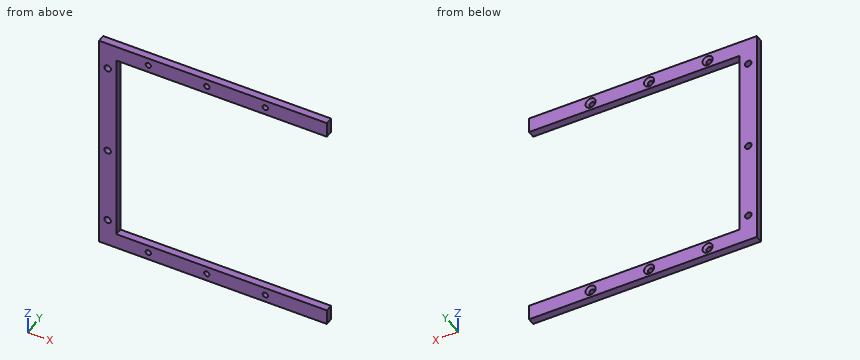
```python
from build123d import *

# Parameters (mm, degrees)
SKETCH2_W           = 7.119984
SKETCH2_H           = 81.28
SKETCH2_R           = 1.35
SKETCH2_W_2         = 93.98
SKETCH2_H_2         = 6.35
SKETCH2_R_2         = 1.1
BOSS_EXTRUDE1_DEPTH = 3
CHAMFER1_SIZE       = 1


with BuildPart() as part:
    # Sketch2 → Boss-Extrude1 (new body)
    # profile 1 of 3: a face of its own
    with BuildSketch(Plane(origin=(0, 0, 0), x_dir=(1, 0, 0), z_dir=(0, 1, 0))):
        with Locations((3.559992, -46.99)):
            Rectangle(SKETCH2_W, SKETCH2_H)
        with Locations(Location((3.559992, -82.490012, 0), (0, 0, 270))):
            Circle(SKETCH2_R, mode=Mode.SUBTRACT)
        with Locations(Location((3.559992, -43.990012, 0), (0, 0, 270))):
            Circle(SKETCH2_R, mode=Mode.SUBTRACT)
        with Locations(Location((3.559992, -11.490012, 0), (0, 0, 270))):
            Circle(SKETCH2_R, mode=Mode.SUBTRACT)
    # profile 2 of 3: a face of its own
    with BuildSketch(Plane(origin=(0, 0, 0), x_dir=(1, 0, 0), z_dir=(0, 1, 0))):
        with Locations((46.99, -3.175)):
            Rectangle(SKETCH2_W_2, SKETCH2_H_2)
        with Locations(Location((68.58, -3.155, 0), (0, 0, 270))):
            Circle(SKETCH2_R_2, mode=Mode.SUBTRACT)
        with Locations(Location((44.45, -3.155, 0), (0, 0, 270))):
            Circle(SKETCH2_R_2, mode=Mode.SUBTRACT)
        with Locations(Location((20.32, -3.155, 0), (0, 0, 270))):
            Circle(SKETCH2_R_2, mode=Mode.SUBTRACT)
    # profile 3 of 3: a face of its own
    with BuildSketch(Plane(origin=(0, 0, 0), x_dir=(1, 0, 0), z_dir=(0, 1, 0))):
        with Locations((46.99, -90.805)):
            Rectangle(SKETCH2_W_2, SKETCH2_H_2)
        with Locations(Location((68.58, -90.805, 0), (0, 0, 270))):
            Circle(SKETCH2_R_2, mode=Mode.SUBTRACT)
        with Locations(Location((44.45, -90.805, 0), (0, 0, 270))):
            Circle(SKETCH2_R_2, mode=Mode.SUBTRACT)
        with Locations(Location((20.32, -90.805, 0), (0, 0, 270))):
            Circle(SKETCH2_R_2, mode=Mode.SUBTRACT)
    extrude(amount=BOSS_EXTRUDE1_DEPTH)

    # Chamfer1
    chamfer1_edges = [part.edges().sort_by_distance(p)[0] for p in [
        (20.32, 3, 89.705),
        (68.58, 3, 2.055),
        (44.45, 3, 2.055),
        (20.32, 3, 2.055),
        (68.58, 3, 89.705),
        (44.45, 3, 89.705),
    ]]
    chamfer(chamfer1_edges, length=CHAMFER1_SIZE)


solid = part.part
```
Design review of the part built by this model. Coordinates are the model's own, in mm. Coordinates: 2 decimals unless noted, no trailing zeros. Order: outer loops, then holes, each group sorted by start corner. A loop starts at its lowest first (then second) coordinate and runs counter-clockwise, first axis right, second up.
1) Take a section at C-C, the plane x = 20.32. Give the boundary of the cut face in (y, z) (3 decimals), and give its area (3 significant figures).
2) Clearance check with flat-ended pins moving along their axes: pin 1 (1.3 mm diameter, centred on x = 44.45, z = 3.155, fed in from +Y); pin 2 (1 mm diameter, centred on y = 2, z = 36.5, fed in from +X). State where each tip first meets the part, or that it passes through.
3) Take a section at B-B, the plane y = 1.15. State how many separate pieces and enclosed holes the cut face has, and give its area (3 significant figures).
4) Wall thickness on line 1 along Z through (x, y) = (68.58, 0.7) (3 decimals); line 2 along Z through (x, y) = (64, 0.2); line 3 along X through (y, z) = (0.95, 50): over which ranges is each line inside the solid? List them lowest first.
5) Take a section at D-D, the plane z = 73. Give the boundary of the cut face in (x, y).
6) Take a section at A-A, the plane x = 52.5. Give the boundary of the cut face in (y, z), and give its area (3 significant figures).
Returned:
1. outline: (0, 0) - (3, 0) - (3, 1.055) - (2, 2.055) - (0, 2.055) - close; (0, 4.255) - (2, 4.255) - (3, 5.255) - (3, 6.35) - (0, 6.35) - close; (0, 87.63) - (3, 87.63) - (3, 88.705) - (2, 89.705) - (0, 89.705) - close; (0, 91.905) - (2, 91.905) - (3, 92.905) - (3, 93.98) - (0, 93.98) - close
1. area: 22.9 mm2
2. pin 1: passes through
2. pin 2: stops at x = 7.12
3. separate pieces: 1
3. enclosed holes: 9
3. area: 1,730 mm2
4. line 1: z = 0 to 2.055, 4.255 to 6.35, 87.63 to 89.705, 91.905 to 93.98
4. line 2: z = 0 to 6.35, 87.63 to 93.98
4. line 3: x = 0 to 7.12
5. outline: (0, 0) - (7.12, 0) - (7.12, 3) - (0, 3) - close
6. outline: (0, 0) - (3, 0) - (3, 6.35) - (0, 6.35) - close; (0, 87.63) - (3, 87.63) - (3, 93.98) - (0, 93.98) - close
6. area: 38.1 mm2
